```python
from build123d import *

# Parameters (mm, degrees)
F1_DEPTH = 11
F3_DEPTH = 2


with BuildPart() as f1:
    # F0 (on Top) → F1 (new body)
    with BuildSketch(Plane.XY):
        with BuildLine():
            ThreePointArc((-2.8726077003, 1.025), (0, 3.05), (2.8726077003, 1.025))
            Line((2.8726077003, 1.025), (6.4693025126, 1.025))
            ThreePointArc((6.4693025126, 1.025), (0, 6.55), (-6.4693025126, 1.025))
            Line((-6.4693025126, 1.025), (-2.8726077003, 1.025))
        make_face()
    extrude(amount=F1_DEPTH)

    # F2 (on face) → F3 (cut, through all)
    with BuildSketch(Plane.XY.offset(11)):
        with BuildLine():
            Line((2.8726077003, 1.025), (3.866442163, 1.025))
            ThreePointArc((3.866442163, 1.025), (0, 4), (-3.866442163, 1.025))
            Line((-3.866442163, 1.025), (-2.8726077003, 1.025))
            ThreePointArc((-2.8726077003, 1.025), (0, 3.05), (2.8726077003, 1.025))
        make_face()
    extrude(amount=-F3_DEPTH, mode=Mode.SUBTRACT)


solid = f1.part
```
Build history of the part. All positions in model axes, mm. A direction names the side the tool comes from. Give positions to 0.01 mm unless a question says otherwise; leave off trailing zeros. Loops run counter-clockwise (first coordinate to the right, second up) from the corner with the lowest first, then second, coordinate; pieces in that order, holes last. Notation, with made-up numbers: (25, 7.25) - (48, 7.25) arc R20 cw to (48, 35.25) - close; hole circle Ø9 at (23.25, -34.75). An arc over 180 degrees is marked (long way). Use a Markdown table: item, result.
(1) Band-saw the part on D-D (x = 4.5). Give the cut face in (y, z) (3 decimals), and give its area (3 significant figures).
Taken from the geometry:
| item | result |
|---|---|
| outline | (1.025, 0) - (4.759, 0) - (4.759, 11) - (1.025, 11) - close |
| area | 41.1 mm2 |
(2) Band-saw the part on B-B (y = 3.6). Give the cut face in (x, z), and give its area (3 significant figures).
Taken from the geometry:
| item | result |
|---|---|
| outline | (-5.47, 0) - (5.47, 0) - (5.47, 11) - (1.74, 11) - (1.74, 9) - (-1.74, 9) - (-1.74, 11) - (-5.47, 11) - close |
| area | 113 mm2 |
(3) Which spindle directions (+Z, -Z, +X, -X, +Y, -Y) get a long thin tool onto all of the face, cutting with end or side? Do faces 1 (the face through (0, 4, 10)), 2 (the face through (5, 1.025, 5)). Say none if no direction does.
Taken from the geometry:
| item | result |
|---|---|
| face 1 | +Z, -Y |
| face 2 | +Z, -Z, +X, -X, -Y |
(4) Pull direction X, two halves, no side cores. Call faces 3 (the face through (-0.1, 3.2, 9)), 4 (the face through (-5, 1.025, 5)), 5 (the face through (0.13, 6.55, 5.42)): +X half, -X half, draft (parallel to the pull), parting line (faces both ways), or undercut.
Taken from the geometry:
| item | result |
|---|---|
| face 3 | undercut |
| face 4 | draft |
| face 5 | parting line |
(5) Drop flat-ended pins along their axis: pin 1 Ø1 at (y, z) = (4.5, 7) entering from +X; pin 2 Ø1.5 at (x, y) = (0, 2.5) entering from +Z; pin 3 Ø1 at (x, z) = (-1, 5) entering from -Y. Give the stop position or say it passes through.
Taken from the geometry:
| item | result |
|---|---|
| pin 1 | x = 5.19 |
| pin 2 | z = 9 |
| pin 3 | y = 2.66 |
(6) Wall check: line 1 along X through (y, z) = (3.3, 10); line 2 along Z through (x, y) = (-3.25, 2); line 3 along X through (y, z) = (2.55, 9.25). Give the ranges that are in metal, low to high.
Taken from the geometry:
| item | result |
|---|---|
| line 1 | -5.66 to -2.26, 2.26 to 5.66 |
| line 2 | 0 to 9 |
| line 3 | -6.03 to -3.08, 3.08 to 6.03 |
(7) Band-saw the part on A-A (y = 2.3). Give the cut face in (x, z).
Taken from the geometry:
| item | result |
|---|---|
| outline | (-6.13, 0) - (-2, 0) - (-2, 9) - (-3.27, 9) - (-3.27, 11) - (-6.13, 11) - close; (2, 0) - (6.13, 0) - (6.13, 11) - (3.27, 11) - (3.27, 9) - (2, 9) - close |
(8) Band-saw the part on C-C (z = 8). Give the cut face in (x, y) (3 decimals), and give its area (3 significant figures).
Taken from the geometry:
| item | result |
|---|---|
| outline | (-6.469, 1.025) - (-2.873, 1.025) arc R3.05 cw to (2.873, 1.025) - (6.469, 1.025) arc R6.55 ccw to start |
| area | 45.5 mm2 |
